from build123d import *

# Parameters (mm, degrees)
ESQUISSE1_R             = 4
BOSS_EXTRU_1_DEPTH      = 60
ENL_V_MAT_EXTRU_2_DEPTH = 1
R_P_T_PAR_COURBE1_COUNT = 12
ESQUISSE5_R             = 1.5


with BuildPart() as part:
    # Esquisse1 → Boss.-Extru.1 (new body)
    with BuildSketch(Plane(origin=(0, 0, 0), x_dir=(1, 0, 0), z_dir=(0, 1, 0))):
        with Locations(Location((0, 0, 0), (0, 0, 270))):
            Circle(ESQUISSE1_R)
    extrude(amount=BOSS_EXTRU_1_DEPTH)

    # Esquisse4 → Enlèv. mat.-Extru.2 (cut)
    with BuildSketch(Plane.XY):
        with BuildLine():
            Line((4, 27.5), (4, 22.5))
            ThreePointArc((4, 22.5), (2, 25), (4, 27.5))
        make_face()
    enl_v_mat_extru_2 = extrude(amount=-ENL_V_MAT_EXTRU_2_DEPTH, mode=Mode.SUBTRACT)

    # Répét. par courbe1: Enlèv. mat.-Extru.2 ×12 about axis
    r_p_t_par_courbe1_axis = Axis((0, 25, 0), (0, -1, 0))
    for i in range(1, R_P_T_PAR_COURBE1_COUNT):
        add(enl_v_mat_extru_2.rotate(r_p_t_par_courbe1_axis, i * 360 / R_P_T_PAR_COURBE1_COUNT), mode=Mode.SUBTRACT)

    # Enlèvement de matière-Balayage1: sweep along a path in Esquisse3
    with BuildLine(Plane(origin=(0, 25, 0), x_dir=(1, 0, 0), z_dir=(0, 1, 0))) as enl_vement_de_mati_re_balayage1_path:
        CenterArc((0, 0), 4, 0, 360)
    # Esquisse5 → Enlèvement de matière-Balayage1 (sweep, cut)
    with BuildSketch(Plane(origin=(0, 0, 0), x_dir=(0, 0, -1), z_dir=(1, 0, 0))):
        with Locations((-4, 25)):
            Circle(ESQUISSE5_R)
    sweep(path=enl_vement_de_mati_re_balayage1_path.line, mode=Mode.SUBTRACT)


solid = part.part
Design review of the part built by this model. Coordinates are the model's own, in mm. A direction names the side the tool comes from. Round coordinates to 2 decimals unless told otherwise and drop trailing zeros. Loops run counter-clockwise (first coordinate to the right, second up) from the corner with the lowest first, then second, coordinate; pieces in that order, holes last. Notation, with made-up numbers: (5.25, -35) -> (16.25, -35) arc R19 cw to (16.25, -10) -> close; hole circle Ø1 at (34, 21). An arc over 180 degrees is marked (long way). Use one line per item in the form item = value. Start each with the question number.
Q1. Wall thickness on line 1 along Y through (x, z) = (2, -3.25); line 2 along X through (y, z) = (28.5, 0.25); line 3 along Z through (x, y) = (-2, 32.5): over which ranges is each line inside the solid? List them lowest first. Write a range as [from, to].
Q2. Machinability: for faces 1 (the face through (0.5, 25, 2)), 2 (the face through (-1.5, 25, 1.4)), 3 (the face through (2.3, 25, 0)), 4 (the face through (1.17, 25.04, -2.03)), which of the approach directions +Z, -Z, +X, -X, +Y, -Y give a long, thin tool a straight path to every point of the face, cutting with its end or side? Answer none if there is none.
Q3. Draft analysis for pull direction Y (two halves, no side actions). For faces 5 (the face through (0, 0, 0)), 6 (the face through (0, 60, 0)), 7 (the face through (-3.905, 11.586, -0.867)), 8 (the face through (1.17, 25.04, 2.03)), state which applies: +Y half, -Y half, draft (parallel to the pull), parting line (faces both ways), or undercut.
Q4. We need section A-A on y = 15. Give the boundary of the cut face in (x, z).
Q5. For pin 1 Ø2 at (x, y) = (-2.5, 23) entering from -Z; pin 2 Ø1.5 at (y, z) = (24, 3) entering from -X; pin 3 Ø2 at (x, y) = (3.5, 24) entering from -Z, all flat-tipped, find the tip position at first contact; note any pin that passes through.
Calculated:
q1.line_1 = [0, 23.51], [26.49, 60]
q1.line_2 = [-3.99, 3.99]
q1.line_3 = [-3.46, 3.46]
q2.face_1 = +Z
q2.face_2 = none
q2.face_3 = +X
q2.face_4 = -Z
q3.face_5 = -Y half
q3.face_6 = +Y half
q3.face_7 = draft
q3.face_8 = undercut
q4.outline = circle Ø8 at (0, 0)
q5.pin_1 = -3.71
q5.pin_2 = -2.85
q5.pin_3 = -3.01
